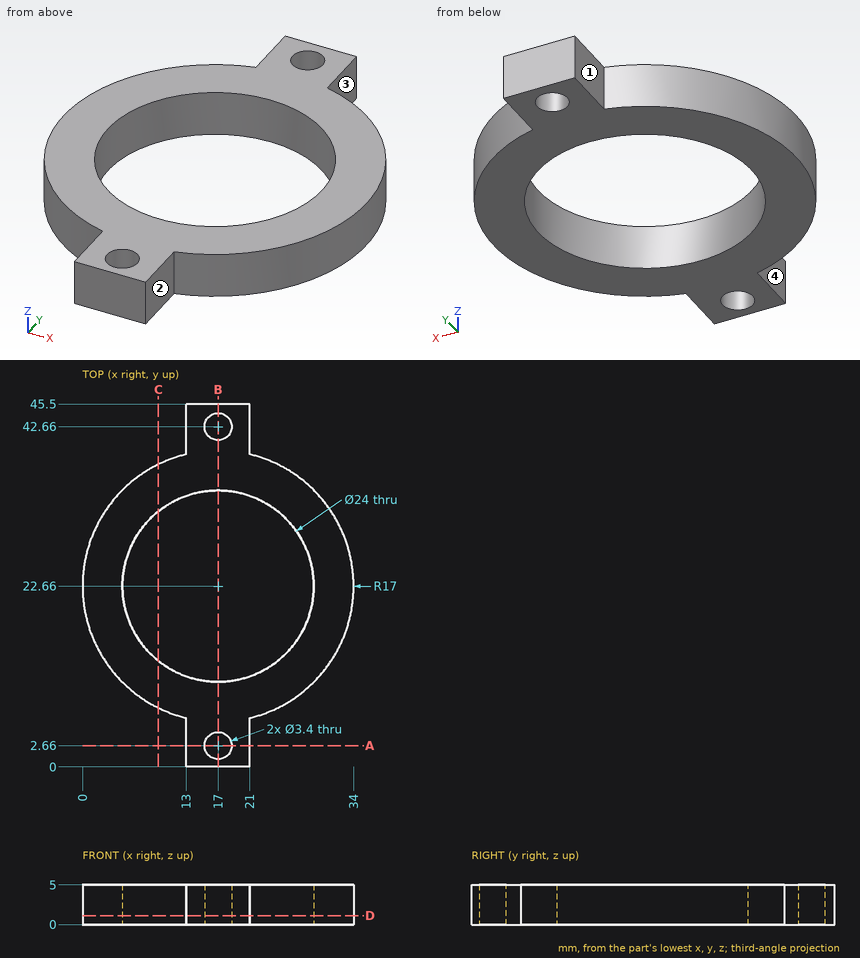
Can you work these out from the drawing? Everything is in mm from the part's minimum corner. A direction names the side the tool comes from. Coordinates: 2 decimals unless noted, no trailing zeros. Loops run counter-clockwise (first coordinate to the right, second up) from the corner with the lowest first, then second, coordinate; pieces in that order, holes last. Notation, with made-up numbers: M 54.5,32.25 L 66.5,32.25 A9 cw 66.5,40.25 Z; hole C 18.25,10.25 d7. An arc over 180 degrees is marked long. Put each result on its own line as item: value. Start each with the question number.
(1) For the marked faces 1, 2, 3 and 4, which set-ups out of +Z, -Z, +X, -X, +Y, -Y let a thin tool reach every point of the face, with its end or its side?
(2) Suppose I cut it at A-A on y = 2.66. Please give me the cut outline in (x, z), then the cut area to 3 significant figures.
(3) Suppose I cut it at B-B on x = 17. Please give me the cut outline in (y, z), then the cut area to 3 significant figures.
(4) I need wall thicknesses on line 1 (Y direction, x = 17, z = 2); line 2 (X direction, y = 42.66, z = 2.05); line 3 (Y direction, x = 16, z = 2.35). Which ranges of each line are inside material? Lowest first, please. Write a range as from..to.
(5) Will these pins go through, and if not, where does the flat tip stop? P1, Ø2, axis at x = 8, y = 29.5, coming from the -Z side; P2, Ø1.5, axis at y = 42.5, z = 1.5, coming from the -X side; P3, Ø2, axis at y = 10.5, z = 1, coming from the +X side.
(6) Suppose I cut it at C-C on x = 9.5. Please give me the cut outline in (y, z).
(7) Suppose I cut it at D-D on z = 1.15. Please give me the cut outline in (x, y).
Solutions:
1. face 1: +Z, -Z, -X, +Y
1. face 2: +Z, -Z, +X, -Y
1. face 3: +Z, -Z, +X, +Y
1. face 4: +Z, -Z, -X, -Y
2. outline: M 13,0 L 15.3,0 L 15.3,5 L 13,5 Z; M 18.7,0 L 21,0 L 21,5 L 18.7,5 Z
2. area: 23.0 mm2
3. outline: M 0,0 L 0.96,0 L 0.96,5 L 0,5 Z; M 4.36,0 L 10.66,0 L 10.66,5 L 4.36,5 Z; M 34.66,0 L 40.96,0 L 40.96,5 L 34.66,5 Z; M 44.36,0 L 45.5,0 L 45.5,5 L 44.36,5 Z
3. area: 73.5 mm2
4. line 1: y = 0..0.96, 4.36..10.66, 34.66..40.96, 44.36..45.5
4. line 2: x = 13..15.3, 18.7..21
4. line 3: y = 0..1.29, 4.03..10.7, 34.62..41.29, 44.03..45.5
5. P1: stops at z = 0
5. P2: stops at x = 13
5. P3: stops at x = 29.82
6. outline: M 7.4,0 L 13.29,0 L 13.29,5 L 7.4,5 Z; M 32.03,0 L 37.92,0 L 37.92,5 L 32.03,5 Z
7. outline: M 13,0 L 21,0 L 21,6.14 A17 ccw 21,39.18 L 21,45.5 L 13,45.5 L 13,39.18 A17 ccw 13,6.14 Z; hole C 17,22.66 d24; hole C 17,2.66 d3.4; hole C 17,42.66 d3.4
